Here's how the part is built. I have some questions about the finished solid (model axes, mm). A direction names the side the tool comes from. Round coordinates to 2 decimals unless told otherwise and drop trailing zeros. Order: outer loops, then holes, each group sorted by start corner. A loop starts at its lowest first (then second) coordinate and runs counter-clockwise, first axis right, second up. Notation, with made-up numbers: (55.25, -23) -> (78.25, -23) arc R24 ccw to (78.25, 13) -> close; hole circle Ø2 at (-7, 30). An arc over 180 degrees is marked (long way). Use a Markdown table: item, result. Add a question column.
(1) If I drill on probe 1 along Z at (x, y) = (8.5, 0.35); probe 2 along X at (y, z) = (-0.4, 36.5); probe 3 along X at (y, z) = (-0.7, 26), over which ranges is the centre line in solid material (lowest first)?
(2) I'm going to push flat-ended pins straight in: P1, Ø0.8, axis at x = 11.5, y = 0.5, coming from the -Z side; P2, Ø8, axis at x = 6.5, z = 29.5, coming from the -Y side; P3, Ø1.2, axis at y = 0, z = 2.5, coming from the +X side. Where does each tip first touch, or does it pass through?
(3) Thinking about a two-plate mould opening in X: for faces 4 (the face through (11, 0, 34)), 5 (the face through (6.57, -0.02, 2.6)), 6 (the face through (16, 0, 8)), which applies, pulls with the +X half, pulls with the -X half, needs draft (parallel to the pull), parting line crosses it, or undercut?
(4) I want a section at A-A, the plane z = 5. Please give me the cut outline in (x, y), then the cut area to 3 significant figures.
(5) I want a section at D-D, the plane z = 31. Please give me the cut outline in (x, y).
(6) I want a section at C-C, the plane y = 0.65. Please give me the cut outline in (x, z), then the cut area to 3 significant figures.
(7) I want a section at B-B, the plane x = 4. Please give me the cut outline in (y, z).
(8) On a 3-axis mill with a long thin cutter (end or side, diameter ignored), from which of +Z, -Z, +X, -X, +Y, -Y can I reach the whole of each face in a straight line? I mean faces 1 (the face through (6, 0, 37)), 2 (the face through (11, 0, 2)), 3 (the face through (15.4, -0.02, 34.57)). Say none if no direction works.
from build123d import *

# Parameters (mm, degrees)
F1_W     = 3
F1_H     = 12.5
F2_DEPTH = 1.25


with BuildPart() as f2:
    # F1 (on Front) → F2 (new body, symmetric)
    with BuildSketch(Plane.XZ):
        Polygon((3, 50), (0, 50), (0, 0), (3, 0), (3, 5.5), (3, 18), (3, 37.5), align=None)
        with Locations((4.5, 43.75)):
            Rectangle(F1_W, F1_H)
        with BuildLine():
            Line((11, 50), (6, 50))
            Line((6, 50), (6, 37.5))
            Line((6, 37.5), (6, 36))
            ThreePointArc((6, 36), (6.5857864376, 34.5857864376), (8, 34))
            Line((8, 34), (14, 34))
            ThreePointArc((14, 34), (15.4142135624, 34.5857864376), (16, 36))
            Line((16, 36), (16, 45))
            ThreePointArc((16, 45), (14.5355339059, 48.5355339059), (11, 50))
        make_face()
        with Locations((4.5, 11.75)):
            Rectangle(F1_W, F1_H)
        with BuildLine():
            Line((11, 18), (6, 18))
            Line((6, 18), (6, 5.5))
            Line((6, 5.5), (6, 4))
            ThreePointArc((6, 4), (6.5857864376, 2.5857864376), (8, 2))
            Line((8, 2), (14, 2))
            ThreePointArc((14, 2), (15.4142135624, 2.5857864376), (16, 4))
            Line((16, 4), (16, 13))
            ThreePointArc((16, 13), (14.5355339059, 16.5355339059), (11, 18))
        make_face()
    extrude(amount=F2_DEPTH, both=True)


solid = f2.part
Taken from the geometry:
| question | item | result |
|---|---|---|
| 1 | probe 1 | z = 2 to 18, 34 to 50 |
| 1 | probe 2 | x = 0 to 3, 6 to 16 |
| 1 | probe 3 | x = 0 to 3 |
| 2 | P1 | stops at z = 2 |
| 2 | P2 | stops at y = -1.25 |
| 2 | P3 | stops at x = 15.79 |
| 3 | face 4 | needs draft |
| 3 | face 5 | undercut |
| 3 | face 6 | pulls with the +X half |
| 4 | outline | (0, -1.25) -> (3, -1.25) -> (3, 1.25) -> (0, 1.25) -> close; (6, -1.25) -> (16, -1.25) -> (16, 1.25) -> (6, 1.25) -> close |
| 4 | area | 32.5 mm2 |
| 5 | outline | (0, -1.25) -> (3, -1.25) -> (3, 1.25) -> (0, 1.25) -> close |
| 6 | outline | (0, 0) -> (3, 0) -> (3, 5.5) -> (6, 5.5) -> (6, 4) arc R2 ccw to (8, 2) -> (14, 2) arc R2 ccw to (16, 4) -> (16, 13) arc R5 ccw to (11, 18) -> (3, 18) -> (3, 37.5) -> (6, 37.5) -> (6, 36) arc R2 ccw to (8, 34) -> (14, 34) arc R2 ccw to (16, 36) -> (16, 45) arc R5 ccw to (11, 50) -> (0, 50) -> close |
| 6 | area | 531 mm2 |
| 7 | outline | (-1.25, 5.5) -> (1.25, 5.5) -> (1.25, 18) -> (-1.25, 18) -> close; (-1.25, 37.5) -> (1.25, 37.5) -> (1.25, 50) -> (-1.25, 50) -> close |
| 8 | face 1 | +Y, -Y |
| 8 | face 2 | -Z, +X, +Y, -Y |
| 8 | face 3 | +X, +Y, -Y |
